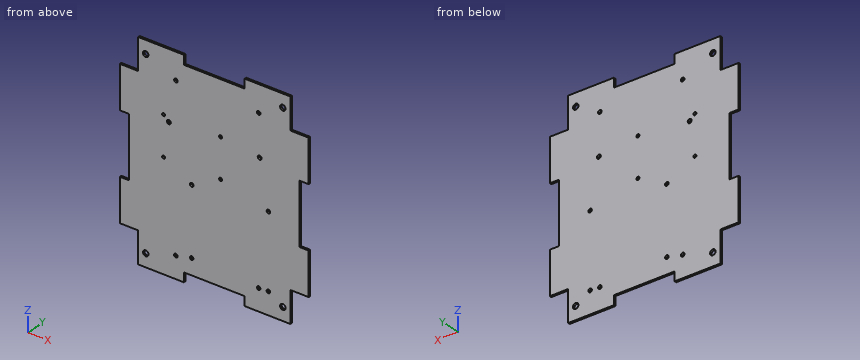
from build123d import *

# Parameters (mm, degrees)
SKETCH1_R          = 2.286
MAIN_BODY_DEPTH    = 1.5875
CUT_EXTRUDE3_REACH = 3.587
SKETCH12_R         = 1.5
SKETCH12_R_2       = 1.25
CUT_EXTRUDE4_REACH = 3.587
SKETCH13_R         = 1.5
SKETCH13_R_2       = 1.625


with BuildPart() as part:
    # Sketch1 → Main Body (new body)
    with BuildSketch(Plane(origin=(0, 0, 0), x_dir=(1, 0, 0), z_dir=(0, 1, 0))):
        Polygon((-25.4, 86.995), (-63.43142, 86.995), (-63.43142, 60.96), (-78.74, 60.96), (-78.74, 25.4), (-71.12, 25.4), (-71.12, -25.4), (-78.74, -25.4), (-78.74, -60.96), (-63.43142, -60.96), (-63.43142, -86.995), (-25.4, -86.995), (-25.4, -79.375), (25.4, -79.375), (25.4, -86.995), (63.43142, -86.995), (63.43142, -60.96), (78.74, -60.96), (78.74, -25.4), (71.12, -25.4), (71.12, 25.4), (78.74, 25.4), (78.74, 60.96), (63.43142, 60.96), (63.43142, 86.995), (25.4, 86.995), (25.4, 79.375), (-25.4, 79.375), align=None)
        with Locations((-57.15, 76.2)):
            Circle(SKETCH1_R, mode=Mode.SUBTRACT)
        with Locations((57.15, 76.2)):
            Circle(SKETCH1_R, mode=Mode.SUBTRACT)
        with Locations((57.15, -76.2)):
            Circle(SKETCH1_R, mode=Mode.SUBTRACT)
        with Locations((-57.15, -76.2)):
            Circle(SKETCH1_R, mode=Mode.SUBTRACT)
    extrude(amount=MAIN_BODY_DEPTH)

    # Sketch12 → Cut-Extrude3 (cut, up to next)
    with BuildSketch(Plane.XZ, mode=Mode.PRIVATE) as cut_extrude3_sk1:
        with Locations((-32, -69)):
            Circle(SKETCH12_R)
    cut_extrude3_tool1 = extrude(cut_extrude3_sk1.sketch, amount=-CUT_EXTRUDE3_REACH, mode=Mode.PRIVATE) & part.part
    add(cut_extrude3_tool1.solids().sort_by_distance((-32, 0, -69))[0], mode=Mode.SUBTRACT)
    # Sketch12 → Cut-Extrude3 (cut, up to next)
    with BuildSketch(Plane.XZ, mode=Mode.PRIVATE) as cut_extrude3_sk2:
        with Locations((37, -69)):
            Circle(SKETCH12_R)
    cut_extrude3_tool2 = extrude(cut_extrude3_sk2.sketch, amount=-CUT_EXTRUDE3_REACH, mode=Mode.PRIVATE) & part.part
    add(cut_extrude3_tool2.solids().sort_by_distance((37, 0, -69))[0], mode=Mode.SUBTRACT)
    # Sketch12 → Cut-Extrude3 (cut, up to next)
    with BuildSketch(Plane.XZ, mode=Mode.PRIVATE) as cut_extrude3_sk3:
        with Locations((37, 65)):
            Circle(SKETCH12_R)
    cut_extrude3_tool3 = extrude(cut_extrude3_sk3.sketch, amount=-CUT_EXTRUDE3_REACH, mode=Mode.PRIVATE) & part.part
    add(cut_extrude3_tool3.solids().sort_by_distance((37, 0, 65))[0], mode=Mode.SUBTRACT)
    # Sketch12 → Cut-Extrude3 (cut, up to next)
    with BuildSketch(Plane.XZ, mode=Mode.PRIVATE) as cut_extrude3_sk4:
        with Locations((-32, 65)):
            Circle(SKETCH12_R)
    cut_extrude3_tool4 = extrude(cut_extrude3_sk4.sketch, amount=-CUT_EXTRUDE3_REACH, mode=Mode.PRIVATE) & part.part
    add(cut_extrude3_tool4.solids().sort_by_distance((-32, 0, 65))[0], mode=Mode.SUBTRACT)
    # Sketch12 → Cut-Extrude3 (cut, up to next)
    with BuildSketch(Plane.XZ, mode=Mode.PRIVATE) as cut_extrude3_sk5:
        with Locations((-42.25, 2.75)):
            Circle(SKETCH12_R_2)
    cut_extrude3_tool5 = extrude(cut_extrude3_sk5.sketch, amount=-CUT_EXTRUDE3_REACH, mode=Mode.PRIVATE) & part.part
    add(cut_extrude3_tool5.solids().sort_by_distance((-42.25, 0, 2.75))[0], mode=Mode.SUBTRACT)
    # Sketch12 → Cut-Extrude3 (cut, up to next)
    with BuildSketch(Plane.XZ, mode=Mode.PRIVATE) as cut_extrude3_sk6:
        with Locations((-42.25, 35.25)):
            Circle(SKETCH12_R_2)
    cut_extrude3_tool6 = extrude(cut_extrude3_sk6.sketch, amount=-CUT_EXTRUDE3_REACH, mode=Mode.PRIVATE) & part.part
    add(cut_extrude3_tool6.solids().sort_by_distance((-42.25, 0, 35.25))[0], mode=Mode.SUBTRACT)
    # Sketch12 → Cut-Extrude3 (cut, up to next)
    with BuildSketch(Plane.XZ, mode=Mode.PRIVATE) as cut_extrude3_sk7:
        with Locations((5.25, 2.75)):
            Circle(SKETCH12_R_2)
    cut_extrude3_tool7 = extrude(cut_extrude3_sk7.sketch, amount=-CUT_EXTRUDE3_REACH, mode=Mode.PRIVATE) & part.part
    add(cut_extrude3_tool7.solids().sort_by_distance((5.25, 0, 2.75))[0], mode=Mode.SUBTRACT)
    # Sketch12 → Cut-Extrude3 (cut, up to next)
    with BuildSketch(Plane.XZ, mode=Mode.PRIVATE) as cut_extrude3_sk8:
        with Locations((5.25, 35.25)):
            Circle(SKETCH12_R_2)
    cut_extrude3_tool8 = extrude(cut_extrude3_sk8.sketch, amount=-CUT_EXTRUDE3_REACH, mode=Mode.PRIVATE) & part.part
    add(cut_extrude3_tool8.solids().sort_by_distance((5.25, 0, 35.25))[0], mode=Mode.SUBTRACT)

    # Sketch13 → Cut-Extrude4 (cut, up to next)
    with BuildSketch(Plane(origin=(0, 1.5875, 0), x_dir=(1, 0, 0), z_dir=(0, 1, 0)), mode=Mode.PRIVATE) as cut_extrude4_sk1:
        with Locations((45.16, 7.6)):
            Circle(SKETCH13_R)
    cut_extrude4_tool1 = extrude(cut_extrude4_sk1.sketch, amount=-CUT_EXTRUDE4_REACH, mode=Mode.PRIVATE) & part.part
    add(cut_extrude4_tool1.solids().sort_by_distance((45.16, 1.5875, -7.6))[0], mode=Mode.SUBTRACT)
    # Sketch13 → Cut-Extrude4 (cut, up to next)
    with BuildSketch(Plane(origin=(0, 1.5875, 0), x_dir=(1, 0, 0), z_dir=(0, 1, 0)), mode=Mode.PRIVATE) as cut_extrude4_sk2:
        with Locations((45.16, 68.6)):
            Circle(SKETCH13_R)
    cut_extrude4_tool2 = extrude(cut_extrude4_sk2.sketch, amount=-CUT_EXTRUDE4_REACH, mode=Mode.PRIVATE) & part.part
    add(cut_extrude4_tool2.solids().sort_by_distance((45.16, 1.5875, -68.6))[0], mode=Mode.SUBTRACT)
    # Sketch13 → Cut-Extrude4 (cut, up to next)
    with BuildSketch(Plane(origin=(0, 1.5875, 0), x_dir=(1, 0, 0), z_dir=(0, 1, 0)), mode=Mode.PRIVATE) as cut_extrude4_sk3:
        with Locations((-18.84, 66.1)):
            Circle(SKETCH13_R)
    cut_extrude4_tool3 = extrude(cut_extrude4_sk3.sketch, amount=-CUT_EXTRUDE4_REACH, mode=Mode.PRIVATE) & part.part
    add(cut_extrude4_tool3.solids().sort_by_distance((-18.84, 1.5875, -66.1))[0], mode=Mode.SUBTRACT)
    # Sketch13 → Cut-Extrude4 (cut, up to next)
    with BuildSketch(Plane(origin=(0, 1.5875, 0), x_dir=(1, 0, 0), z_dir=(0, 1, 0)), mode=Mode.PRIVATE) as cut_extrude4_sk4:
        with Locations((-18.84, 10.1)):
            Circle(SKETCH13_R)
    cut_extrude4_tool4 = extrude(cut_extrude4_sk4.sketch, amount=-CUT_EXTRUDE4_REACH, mode=Mode.PRIVATE) & part.part
    add(cut_extrude4_tool4.solids().sort_by_distance((-18.84, 1.5875, -10.1))[0], mode=Mode.SUBTRACT)
    # Sketch13 → Cut-Extrude4 (cut, up to next)
    with BuildSketch(Plane(origin=(0, 1.5875, 0), x_dir=(1, 0, 0), z_dir=(0, 1, 0)), mode=Mode.PRIVATE) as cut_extrude4_sk5:
        with Locations((-37.85, -31.1)):
            Circle(SKETCH13_R_2)
    cut_extrude4_tool5 = extrude(cut_extrude4_sk5.sketch, amount=-CUT_EXTRUDE4_REACH, mode=Mode.PRIVATE) & part.part
    add(cut_extrude4_tool5.solids().sort_by_distance((-37.85, 1.5875, 31.1))[0], mode=Mode.SUBTRACT)
    # Sketch13 → Cut-Extrude4 (cut, up to next)
    with BuildSketch(Plane(origin=(0, 1.5875, 0), x_dir=(1, 0, 0), z_dir=(0, 1, 0)), mode=Mode.PRIVATE) as cut_extrude4_sk6:
        with Locations((37.85, -31.1)):
            Circle(SKETCH13_R_2)
    cut_extrude4_tool6 = extrude(cut_extrude4_sk6.sketch, amount=-CUT_EXTRUDE4_REACH, mode=Mode.PRIVATE) & part.part
    add(cut_extrude4_tool6.solids().sort_by_distance((37.85, 1.5875, 31.1))[0], mode=Mode.SUBTRACT)


solid = part.part
The listing builds one solid part. Answer for the finished solid, in the listing's coordinates (mm). Coordinates: 2 decimals unless noted, no trailing zeros. Loops run counter-clockwise (first coordinate to the right, second up) from the corner with the lowest first, then second, coordinate; pieces in that order, holes last.
1) Find section C-C on y = 0.55. Give the number of separate pieces and of enclosed holes in the cut face, then the cut area to 3 significant figures.
2) Find the intervals of material crossed by L1, parallel to X at y = 0.45, z = 76.2; L2, parallel to Z at x = 5.25, y = 0.7 (3 decimals); L3, parallel to Z at x = 45.16, y = 1.35 (3 decimals), in increasing order.
3) Flat-ended cylindrical pins translate along their axes: pin 1 Ø3.5 at (x, z) = (37, 65) entering from -Y; pin 2 Ø0.8 at (x, y) = (71, 1) entering from +Z; pin 3 Ø0.8 at (y, z) = (0.5, -83) entering from +X; pin 4 Ø0.5 at (x, y) = (-8, 0.5) entering from +Z (3 decimals). Find the tip coordinate at first contact, or state that the pin passes through.
4) Find section A-A on x = -57.15. Write down the section's boundary in (y, z) (1 decimal).
5) Find section D-D on x = -13. Write down the section's boundary in (y, z) (1 decimal), then the cut area to 3 significant figures.
6) Find section B-B on z = 76.2. Write down the section's boundary in (x, y), then the cut area to 3 significant figures.
Values:
1. separate pieces: 1
1. enclosed holes: 18
1. area: 24,100 mm2
2. L1: x = -63.43 to -59.44, -54.86 to 54.86, 59.44 to 63.43
2. L2: z = -79.375 to 1.5, 4 to 34, 36.5 to 79.375
2. L3: z = -86.995 to -70.1, -67.1 to -9.1, -6.1 to 86.995
3. pin 1: stops at y = 0
3. pin 2: stops at z = 60.96
3. pin 3: stops at x = 63.43
3. pin 4: stops at z = 79.375
4. outline: (0, -87) - (1.6, -87) - (1.6, -78.5) - (0, -78.5) - close; (0, -73.9) - (1.6, -73.9) - (1.6, 73.9) - (0, 73.9) - close; (0, 78.5) - (1.6, 78.5) - (1.6, 87) - (0, 87) - close
5. outline: (0, -79.4) - (1.6, -79.4) - (1.6, 79.4) - (0, 79.4) - close
5. area: 252 mm2
6. outline: (-63.43, 0) - (-59.44, 0) - (-59.44, 1.59) - (-63.43, 1.59) - close; (-54.86, 0) - (54.86, 0) - (54.86, 1.59) - (-54.86, 1.59) - close; (59.44, 0) - (63.43, 0) - (63.43, 1.59) - (59.44, 1.59) - close
6. area: 187 mm2
